Source: CAD feature listing. Evaluate the final solid. Frame: model axes, mm. Coordinates: 2 decimals unless noted, no trailing zeros. Order: outer loops, then holes, each group sorted by start corner. A loop starts at its lowest first (then second) coordinate and runs counter-clockwise, first axis right, second up.
```python
from build123d import *

# Parameters (mm, degrees)
F0_R          = 15.875
F1_DEPTH      = 101.6
F1_DEPTH_BACK = 12.7
F2_SIZE       = 1.5875
F3_SIZE       = 3.175
F5_START      = -4.7625
F5_DEPTH      = 9.4488


with BuildPart() as f1:
    # F0 (on Front) → F1 (new body, two sides)
    with BuildSketch(Plane.XZ) as f1_sk:
        Circle(F0_R)
    extrude(amount=F1_DEPTH)
    extrude(f1_sk.sketch, amount=-F1_DEPTH_BACK)

    # F2
    f2_edges = [f1.edges().sort_by_distance(p)[0] for p in [
        (-15.875, -101.6, 0),
    ]]
    chamfer(f2_edges, length=F2_SIZE)

    # F3
    f3_edges = [f1.edges().sort_by_distance(p)[0] for p in [
        (-15.875, 12.7, 0),
    ]]
    chamfer(f3_edges, length=F3_SIZE)

    # F4 (on face) → F5 (cut)
    with BuildSketch(Plane.XZ.offset(101.6).offset(F5_START)):
        with BuildLine():
            Line((0, 14.2875), (6.9197520729, 14.2875))
            ThreePointArc((6.9197520729, 14.2875), (0, 15.875), (-6.9197520729, 14.2875))
            Line((-6.9197520729, 14.2875), (0, 14.2875))
        make_face()
    extrude(amount=-F5_DEPTH, mode=Mode.SUBTRACT)


solid = f1.part
```
1. Draft query along Y for faces 1 (the face through (0, -101.6, 0)), 2 (the face through (0, -92, 14.288)), 3 (the face through (5.93, 12.55, -11.4)). Return one class per face: released by +Y, released by -Y, zero draft, split by the parting line, or undercut.
Findings:
face 1: released by -Y
face 2: undercut
face 3: released by +Y
2. Pin query (flat end, axial travel): P1, Ø12, axis at y = -7.5, z = 10, coming from the -X side; P2, Ø4.5, axis at x = 1.5, y = -94, coming from the +Z side; P3, Ø1, axis at x = -9.5, y = -52, coming from the -Z side. Return the tip coordinate at first contact, or that it passes through.
Findings:
P1: stops at x = -15.36
P2: stops at z = 14.29
P3: stops at z = -13.08
3. Section query A-A on y = -2.5. Return loops of the section in (x, z) (3 decimals), plus the area to 3 significant figures.
Findings:
outline: circle Ø31.75 at (0, 0)
area: 792 mm2
4. Ray query, line 1 (Z direction, x = -6, y = -16); line 2 (Z direction, x = 7, y = -66.5). Return the intervals inside material, ascending.
Findings:
line 1: z = -14.7 to 14.7
line 2: z = -14.25 to 14.25
